Could you check a few things on this model? Use its own coordinates, in mm. Face numbers are marked on the shaded views. Coordinates: 2 decimals unless noted, no trailing zeros. Loops run counter-clockwise (first coordinate to the right, second up) from the corner with the lowest first, then second, coordinate; pieces in that order, holes last. Notation, with made-up numbers: (37.25, -33.75) - (61.25, -33.75) arc R29 cw to (61.25, 3.25) - close; hole circle Ø1 at (57.25, 74). An arc over 180 degrees is marked (long way). Use CSV: the item, a comma, the result in double quotes.
from build123d import *

# Parameters (mm, degrees)
SKETCH1_W                   = 60
SKETCH1_H                   = 36.5
BOSS_EXTRUDE1_DEPTH         = 10
SKETCH2_W                   = 60
SKETCH2_H                   = 5
CUT_EXTRUDE1_DEPTH          = 5
TAP_DRILL_FOR_M5_TAP1_D     = 5.2
TAP_DRILL_FOR_M5_TAP1_DEPTH = 46
TAP_DRILL_FOR_M5_TAP1_TIP   = 1.562237609


with BuildPart() as part:
    # Sketch1 → Boss-Extrude1 (new body)
    with BuildSketch(Plane(origin=(0, 0, 0), x_dir=(1, 0, 0), z_dir=(0, 1, 0))):
        Rectangle(SKETCH1_W, SKETCH1_H)
    extrude(amount=BOSS_EXTRUDE1_DEPTH)

    # Sketch2 → Cut-Extrude1 (cut)
    with BuildSketch(Plane(origin=(0, 10, 0), x_dir=(1, 0, 0), z_dir=(0, 1, 0))):
        with Locations((0, -15.75)):
            Rectangle(SKETCH2_W, SKETCH2_H)
    extrude(amount=-CUT_EXTRUDE1_DEPTH, mode=Mode.SUBTRACT)

    # Tap Drill for M5 Tap1
    with Locations(Plane(origin=(-15, 10, 0), x_dir=(0, 0, 1), z_dir=(0, 1, 0))):
        with Locations((0, 0), (0, 30)):
            Hole(TAP_DRILL_FOR_M5_TAP1_D / 2, depth=TAP_DRILL_FOR_M5_TAP1_DEPTH)
            with Locations((0, 0, -(TAP_DRILL_FOR_M5_TAP1_DEPTH + TAP_DRILL_FOR_M5_TAP1_TIP / 2))):  # 118° drill point
                Cone(0, TAP_DRILL_FOR_M5_TAP1_D / 2, TAP_DRILL_FOR_M5_TAP1_TIP, mode=Mode.SUBTRACT)


solid = part.part
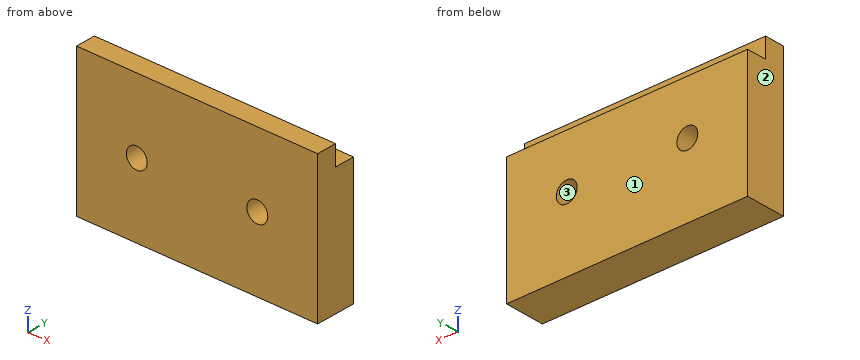
(1) Thinking about a two-plate mould opening in X: for the marked faces 1, 2 and 3, which applies, +X half, -X half, draft (parallel to the pull), parting line (faces both ways), or undercut?
Computed:
face 1,"draft"
face 2,"-X half"
face 3,"undercut"
(2) Suppose I cut it at D-D (x = 1). Write out the boundary of the cut face in (y, z).
Computed:
outline,"(0, -18.25) - (10, -18.25) - (10, 13.25) - (5, 13.25) - (5, 18.25) - (0, 18.25) - close"
(3) Suppose I cut it at C-C (y = 6). Write out the boundary of the cut face in (x, z).
Computed:
outline,"(-30, -18.25) - (30, -18.25) - (30, 13.25) - (-30, 13.25) - close; hole circle Ø5.2 at (-15, 0); hole circle Ø5.2 at (15, 0)"
(4) Please list where these lines run through material, in increasing order: line 1 (X direction, y = 5.5, z = 0); line 2 (Z direction, x = -10, y = 7); line 3 (Z direction, x = 17, y = 5.25).
Computed:
line 1,"x = -30 to -17.6, -12.4 to 12.4, 17.6 to 30"
line 2,"z = -18.25 to 13.25"
line 3,"z = -18.25 to -1.66, 1.66 to 13.25"
(5) Suppose I cut it at B-B (z = 1). Write out the boundary of the cut face in (x, y).
Computed:
outline,"(-30, 0) - (-17.4, 0) - (-17.4, 10) - (-30, 10) - close; (-12.6, 0) - (12.6, 0) - (12.6, 10) - (-12.6, 10) - close; (17.4, 0) - (30, 0) - (30, 10) - (17.4, 10) - close"
(6) Suppose I cut it at A-A (x = 15). Write out the boundary of the cut face in (y, z).
Computed:
outline,"(0, -18.25) - (10, -18.25) - (10, -2.6) - (0, -2.6) - close; (0, 2.6) - (10, 2.6) - (10, 13.25) - (5, 13.25) - (5, 18.25) - (0, 18.25) - close"
(7) Will this pin go through, and if not, where does the flat tip stop? pin 1 (1.5 mm diameter, centred on x = 12, z = 16, fed in from +Y).
Computed:
pin 1,"stops at y = 5"
